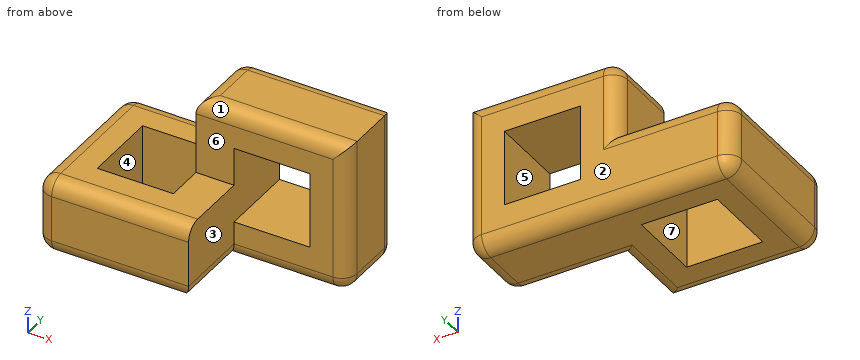
from build123d import *

# Parameters (mm, degrees)
F0_W     = 35
F0_H     = 20
F0_W_2   = 10
F0_H_2   = 10
F1_DEPTH = 20
F2_W     = 10
F2_H     = 5
F3_DEPTH = 25
F5_DEPTH = 10
F6_DEPTH = 10
F7_R     = 2


with BuildPart() as f1:
    # F0 (on Top) → F1 (new body)
    with BuildSketch(Plane.XY):
        with Locations((12.5, 5)):
            Rectangle(F0_W, F0_H)
        with Locations((5, 5)):
            Rectangle(F0_W_2, F0_H_2, mode=Mode.SUBTRACT)
    extrude(amount=F1_DEPTH)

    # F2 (on face) → F3 (cut)
    with BuildSketch(Plane.XZ.offset(5)):
        with Locations((20, 12.5)):
            Rectangle(F2_W, F2_H)
        with Locations((20, 7.5)):
            Rectangle(F2_W, F2_H)
    extrude(amount=-F3_DEPTH, mode=Mode.SUBTRACT)

    # F4 (on face) → F5 (cut)
    with BuildSketch(Plane.XY.offset(20)):
        Polygon((10, 10), (10, 15), (-5, 15), (-5, -5), (10, -5), (10, 0), (0, 0), (0, 10), align=None)
    extrude(amount=-F5_DEPTH, mode=Mode.SUBTRACT)

    # F2 (on face) → F6 (cut)
    with BuildSketch(Plane.XZ.offset(5)):
        Polygon((15, 10), (15, 15), (25, 15), (25, 10), (30, 10), (30, 20), (10, 20), (10, 10), align=None)
        Polygon((30, 10), (25, 10), (25, 5), (15, 5), (15, 0), (30, 0), align=None)
    extrude(amount=-F6_DEPTH, mode=Mode.SUBTRACT)

    # F7
    f7_edges = [f1.edges().sort_by_distance(p)[0] for p in [
        (-5, 5, 10),
        (5, -5, 10),
        (2.5, 15, 10),
        (10, 15, 15),
        (10, 10, 20),
        (20, 15, 20),
        (30, 15, 10),
        (12.5, 15, 0),
        (-5, 15, 5),
        (-5, -5, 5),
        (30, 10, 0),
        (22.5, 5, 0),
        (15, 0, 0),
        (30, 5, 10),
        (20, 5, 20),
        (5, -5, 0),
        (-5, 5, 0),
    ]]
    fillet(f7_edges, radius=F7_R)


solid = f1.part
CAD build for the part. Positions are in the model's coordinates, mm. Face numbers are marked on the shaded views. A direction names the side the tool comes from. Round coordinates to 2 decimals unless told otherwise and drop trailing zeros. Order: outer loops, then holes, each group sorted by start corner. A loop starts at its lowest first (then second) coordinate and runs counter-clockwise, first axis right, second up. Notation, with made-up numbers: M -28.5,-35 L 3.5,-35 A13 ccw 3.5,-30 Z; hole C 1,26.25 d9. An arc over 180 degrees is marked long. Use one line per item in the form item = value.
Q1. Saw through at D-D on z = 7. Give the cut face in (x, y), then the cut area to 3 significant figures.
Recorded:
outline = M -5,-3 A2 ccw -3,-5 L 15,-5 L 15,15 L -3,15 A2 ccw -5,13 Z; M 25,5 L 28,5 A2 ccw 30,7 L 30,13 A2 ccw 28,15 L 25,15 Z; hole M 0,0 L 10,0 L 10,10 L 0,10 Z
area = 347 mm^2
Q2. Saw through at B-B on z = 14.5. Give the cut face in (x, y).
Recorded:
outline = M 10,5 L 15,5 L 15,15 L 12,15 A2 ccw 10,13 Z; M 25,5 L 28,5 A2 ccw 30,7 L 30,13 A2 ccw 28,15 L 25,15 Z
Q3. Which spindle directions (+Z, -Z, +X, -X, +Y, -Y) get a long thin tool onto all of the face, cutting with end or side? Do the marked faces 5, 6 and 7. Say none if no direction does.
Recorded:
face_5 = +Y, -Y
face_6 = +Z, +X, -Y
face_7 = +Z
Q4. Two-plate mould, pull along Y, no slides. Class the marked faces 1, 2, 3 and 4: +Y half, -Y half, draft (parallel to the pull), parting line (faces both ways), or undercut.
Recorded:
face_1 = -Y half
face_2 = +Y half
face_3 = draft
face_4 = undercut
Q5. Flat gauge pins, fed straight in: P1, Ø5, axis at y = 4, z = 13.5, coming from the -X side; P2, Ø3, axis at y = 12, z = 10, coming from the -X side; P3, Ø1.5, axis at y = 4, z = 17.5, coming from the -X side; P4, Ø6, axis at x = 2, y = 9.5, coming from the -Z side. Where does each tip first touch, or does it go through?
Recorded:
P1 = 10
P2 = -4.94
P3 = through
P4 = 0
Q6. Saw through at A-A on x = 3. Give the cut face in (y, z), then the cut area to 3 significant figures.
Recorded:
outline = M -5,2 A2 ccw -3,0 L 0,0 L 0,10 L -3,10 A2 ccw -5,8 Z; M 10,0 L 13,0 A2 ccw 15,2 L 15,8 A2 ccw 13,10 L 10,10 Z
area = 96.6 mm^2
Q7. Saw through at C-C on y = 6.25. Give the cut face in (x, z), then the cut area to 3 significant figures.
Recorded:
outline = M -5,2 A2 ccw -3,0 L 0,0 L 0,10 L -3,10 A2 ccw -5,8 Z; M 10,0 L 13,0 A2 ccw 13.75,0.15 L 28,0.15 A1.85 ccw 29.85,2 L 29.85,19.85 L 11.25,19.85 A2 ccw 10,18 Z; hole M 15,5 L 25,5 L 25,15 L 15,15 Z
area = 339 mm^2
Q8. Probe L1, parallel to X at y = 9.5, z = 9.5; L2, parallel to X at y = 4.75, z = 4; L3, parallel to X at y = 7.5, z = 12.75. List the from-to ranges inside material, lowest first.
Recorded:
L1 = -4.32 to 0, 10 to 15, 25 to 30
L2 = -5 to 0, 10 to 15
L3 = 10 to 15, 25 to 30
